Read the model definition and answer for the solid it produces. Units are mm, in the model's axes. Coordinates: 2 decimals unless noted, no trailing zeros. Loops run counter-clockwise (first coordinate to the right, second up) from the corner with the lowest first, then second, coordinate; pieces in that order, holes last.
from build123d import *

# Parameters (mm, degrees)
ESQUISSE1_R        = 1.5
ESQUISSE1_R_2      = 8.5
ESQUISSE1_R_3      = 1.25
BOSS_EXTRU_1_DEPTH = 1.5
CONG_1_R           = 5


with BuildPart() as part:
    # Esquisse1 → Boss.-Extru.1 (new body)
    with BuildSketch(Plane(origin=(0, 0, 0), x_dir=(1, 0, 0), z_dir=(0, 1, 0))):
        with BuildLine():
            Line((-150, -35), (150, -35))
            Line((150, -35), (150, -87.757984761))
            ThreePointArc((150, -87.757984761), (134.899573158, -109.560800704), (116.657363934, -128.81196889))
            ThreePointArc((116.657363934, -128.81196889), (99.830836188, -131.749824312), (89.940729359, -117.823273505))
            ThreePointArc((89.940729359, -117.823273505), (49.2602069, -80.006841758), (10.006092194, -119.301903743))
            Line((10.006092194, -119.301903743), (9.546735179, -145.618449467))
            ThreePointArc((9.546735179, -145.618449467), (0, -155), (-9.546735179, -145.618449467))
            Line((-9.546735179, -145.618449467), (-10.006092194, -119.301903743))
            ThreePointArc((-10.006092194, -119.301903743), (-49.2602069, -80.006841758), (-89.940729359, -117.823273505))
            ThreePointArc((-89.940729359, -117.823273505), (-99.830836188, -131.749824312), (-116.657363934, -128.81196889))
            ThreePointArc((-116.657363934, -128.81196889), (-134.899573158, -109.560800704), (-150, -87.757984761))
            Line((-150, -87.757984761), (-150, -35))
        make_face()
        with Locations(Location((-70, -45, 0), (0, 0, 270))):
            Circle(ESQUISSE1_R, mode=Mode.SUBTRACT)
        with Locations(Location((0, -45, 0), (0, 0, 270))):
            Circle(ESQUISSE1_R, mode=Mode.SUBTRACT)
        with Locations(Location((105.917021103, -116.952582907, 0), (0, 0, 90))):
            Circle(ESQUISSE1_R_2, mode=Mode.SUBTRACT)
        with Locations(Location((-105.917021103, -116.952582907, 0), (0, 0, 270))):
            Circle(ESQUISSE1_R_2, mode=Mode.SUBTRACT)
        with Locations(Location((-100.143518411, -106.952582907, 0), (0, 0, 270))):
            Circle(ESQUISSE1_R, mode=Mode.SUBTRACT)
        with Locations(Location((70, -45, 0), (0, 0, 90))):
            Circle(ESQUISSE1_R, mode=Mode.SUBTRACT)
        with Locations(Location((-100.143518411, -126.952582907, 0), (0, 0, 270))):
            Circle(ESQUISSE1_R, mode=Mode.SUBTRACT)
        with Locations(Location((-117.464026487, -116.952582907, 0), (0, 0, 270))):
            Circle(ESQUISSE1_R, mode=Mode.SUBTRACT)
        with Locations(Location((100.143518411, -126.952582907, 0), (0, 0, 90))):
            Circle(ESQUISSE1_R, mode=Mode.SUBTRACT)
        with Locations(Location((117.464026487, -116.952582907, 0), (0, 0, 90))):
            Circle(ESQUISSE1_R, mode=Mode.SUBTRACT)
        with Locations(Location((-140, -45, 0), (0, 0, 270))):
            Circle(ESQUISSE1_R, mode=Mode.SUBTRACT)
        with Locations(Location((140, -45, 0), (0, 0, 90))):
            Circle(ESQUISSE1_R, mode=Mode.SUBTRACT)
        with Locations(Location((100.143518411, -106.952582907, 0), (0, 0, 90))):
            Circle(ESQUISSE1_R, mode=Mode.SUBTRACT)
        with Locations(Location((0, -145.451810585, 0), (0, 0, 270))):
            Circle(ESQUISSE1_R_3, mode=Mode.SUBTRACT)
        with Locations(Location((-60, -75, 0), (0, 0, 270))):
            Circle(ESQUISSE1_R, mode=Mode.SUBTRACT)
        with Locations(Location((-90, -95, 0), (0, 0, 270))):
            Circle(ESQUISSE1_R, mode=Mode.SUBTRACT)
        with Locations(Location((90, -95, 0), (0, 0, 90))):
            Circle(ESQUISSE1_R, mode=Mode.SUBTRACT)
        with Locations(Location((60, -75, 0), (0, 0, 90))):
            Circle(ESQUISSE1_R, mode=Mode.SUBTRACT)
        with Locations(Location((0, -105, 0), (0, 0, 270))):
            Circle(ESQUISSE1_R, mode=Mode.SUBTRACT)
        with Locations(Location((0, -75, 0), (0, 0, 270))):
            Circle(ESQUISSE1_R, mode=Mode.SUBTRACT)
        with Locations(Location((145, -86.810137657, 0), (0, 0, 270))):
            Circle(ESQUISSE1_R, mode=Mode.SUBTRACT)
        with Locations(Location((127.366151897, -111.0804364, 0), (0, 0, 270))):
            Circle(ESQUISSE1_R, mode=Mode.SUBTRACT)
        with Locations(Location((-127.366151897, -111.0804364, 0), (0, 0, 90))):
            Circle(ESQUISSE1_R, mode=Mode.SUBTRACT)
        with Locations(Location((-145, -86.810137657, 0), (0, 0, 90))):
            Circle(ESQUISSE1_R, mode=Mode.SUBTRACT)
    extrude(amount=BOSS_EXTRU_1_DEPTH)

    # Congé1
    cong_1_edges = [part.edges().sort_by_distance(p)[0] for p in [
        (-150, 0.75, 35),
        (150, 0.75, 35),
        (150, 0.75, 87.757984761),
        (-150, 0.75, 87.757984761),
    ]]
    fillet(cong_1_edges, radius=CONG_1_R)


solid = part.part
Item 1: Find the intervals of material crossed by line 1 along X through (y, z) = (0.9, 45); line 2 along X through (y, z) = (1, 127); line 3 along Z through (x, y) = (70, 0.45), in increasing order.
Numbers:
line 1: x = -150 to -141.5, -138.5 to -71.5, -68.5 to -1.5, 1.5 to 68.5, 71.5 to 138.5, 141.5 to 150
line 2: x = -118.63 to -101.64, -98.64 to -93.47, -9.87 to 9.87, 93.47 to 98.64, 101.64 to 118.63
line 3: z = 35 to 43.5, 46.5 to 85.36
Item 2: Determine the mould class of faces 1 (the face through (-99.598, 0.74, 131.652)), 2 (the face through (2, 1.5, 81)), 3 (the face through (100.172, 0.74, 123.217)) for opening direction Z: released by +Z, released by -Z, zero draft, split by the parting line, or undercut.
Numbers:
face 1: released by +Z
face 2: zero draft
face 3: undercut
Item 3: A cutting plane is placed at B-B on x = 50. Determine the outline of the cut face in (y, z).
Numbers:
outline: (0, 35) - (1.5, 35) - (1.5, 80) - (0, 80) - close
Item 4: A cutting plane is placed at A-A on z = 122. Determine the outline of the cut face in (x, y), then the cut area to 3 significant figures.
Numbers:
outline: (-123.76, 0) - (-112.76, 0) - (-112.76, 1.5) - (-123.76, 1.5) - close; (-99.08, 0) - (-90.73, 0) - (-90.73, 1.5) - (-99.08, 1.5) - close; (-9.96, 0) - (9.96, 0) - (9.96, 1.5) - (-9.96, 1.5) - close; (90.73, 0) - (99.08, 0) - (99.08, 1.5) - (90.73, 1.5) - close; (112.76, 0) - (123.76, 0) - (123.76, 1.5) - (112.76, 1.5) - close
area: 87.9 mm2
Item 5: Given pin 1 (3.5 mm diameter, centred on x = -140, z = 45, fed in from +Y), flat-ended and moving along its own axis, determine where the tip first touches the part or whether it passes through.
Numbers:
pin 1: stops at y = 1.5
Item 6: A cutting plane is placed at D-D on x = -48.5. Determine the outline of the cut face in (y, z), then the cut area to 3 significant figures.
Numbers:
outline: (0, 35) - (1.5, 35) - (1.5, 80.03) - (0, 80.03) - close
area: 67.5 mm2
Item 7: A cutting plane is placed at C-C on y = 1.05. Give the number of separate pieces and of enclosed holes in the cut face, then the cut area to 3 significant figures.
Numbers:
separate pieces: 1
enclosed holes: 24
area: 20,400 mm2
